from build123d import *

# Parameters (mm, degrees)
SKETCH1_W           = 65
SKETCH1_H           = 159.8
BOSS_EXTRUDE1_DEPTH = 2.5
SKETCH2_W           = 15
SKETCH2_H           = 30
BOSS_EXTRUDE2_DEPTH = 25
SKETCH3_R           = 5.1
CUT_EXTRUDE1_DEPTH  = 107.607973435
SKETCH6_W           = 5
SKETCH6_H           = 5
BOSS_EXTRUDE4_DEPTH = 5
SKETCH7_R           = 5
BOSS_EXTRUDE5_DEPTH = 21
SKETCH8_R           = 15
BOSS_EXTRUDE6_DEPTH = 3
FILLET1_R           = 1.5
CHAMFER1_SIZE       = 1.5
FILLET2_R           = 1.5


with BuildPart() as part:
    # Sketch1 → Boss-Extrude1 (new, symmetric)
    with BuildSketch(Plane(origin=(0, 0, 0), x_dir=(1, 0, 0), z_dir=(0, 1, 0))):
        Rectangle(SKETCH1_W, SKETCH1_H)
    extrude(amount=BOSS_EXTRUDE1_DEPTH, both=True)

    # Sketch2 → Boss-Extrude2 (add)
    with BuildSketch(Plane(origin=(0, 2.5, 0), x_dir=(1, 0, 0), z_dir=(0, 1, 0))):
        with Locations((-25, 0)):
            Rectangle(SKETCH2_W, SKETCH2_H)
    extrude(amount=BOSS_EXTRUDE2_DEPTH)

    # Sketch3 → Cut-Extrude1 (cut, through all)
    with BuildSketch(Plane.ZY.offset(32.5)):
        with Locations((0, 15)):
            Circle(SKETCH3_R)
    extrude(amount=-CUT_EXTRUDE1_DEPTH, mode=Mode.SUBTRACT)

    # Sketch6 → Boss-Extrude4 (add)
    with BuildSketch(Plane.XZ.offset(2.5)):
        with Locations((30, 77.4)):
            Rectangle(SKETCH6_W, SKETCH6_H)
        with Locations((30, -77.4)):
            Rectangle(SKETCH6_W, SKETCH6_H)
    extrude(amount=BOSS_EXTRUDE4_DEPTH)

    # Sketch7 → Boss-Extrude5 (add)
    with BuildSketch(Plane(origin=(0, 2.5, 0), x_dir=(1, 0, 0), z_dir=(0, 1, 0))):
        with Locations(Location((-11.5, 40, 0), (0, 0, 90))):
            Circle(SKETCH7_R)
        with Locations(Location((-11.5, -40, 0), (0, 0, 90))):
            Circle(SKETCH7_R)
    extrude(amount=BOSS_EXTRUDE5_DEPTH)

    # Sketch8 → Boss-Extrude6 (add)
    with BuildSketch(Plane(origin=(0, 23.5, 0), x_dir=(1, 0, 0), z_dir=(0, 1, 0))):
        with Locations(Location((-11.5, 40, 0), (0, 0, 270))):
            Circle(SKETCH8_R)
        with Locations(Location((-11.5, -40, 0), (0, 0, 90))):
            Circle(SKETCH8_R)
    extrude(amount=BOSS_EXTRUDE6_DEPTH)

    # Fillet1
    fillet1_edges = [part.edges().sort_by_distance(p)[0] for p in [
        (-11.5, 23.5, -55),
        (-11.5, 26.5, -55),
        (-11.5, 23.5, 55),
        (-11.5, 26.5, 55),
    ]]
    fillet(fillet1_edges, radius=FILLET1_R - 0.0001)  # a hair under: the kernel refuses the full size

    # Chamfer1
    chamfer1_edges = [part.edges().sort_by_distance(p)[0] for p in [
        (-32.5, 15, -5.1),
    ]]
    chamfer(chamfer1_edges, length=CHAMFER1_SIZE)

    # Fillet2
    fillet2_edges = [part.edges().sort_by_distance(p)[0] for p in [
        (-32.5, 15, -15),
        (-32.5, 15, 15),
        (-17.5, 15, 15),
        (-17.5, 15, -15),
        (-32.5, 27.5, 0),
        (-25, 27.5, 15),
        (-17.5, 27.5, 0),
        (-25, 27.5, -15),
    ]]
    fillet(fillet2_edges, radius=FILLET2_R)


solid = part.part
Can you work these out from the model? Positions are in its coordinate system, mm. A direction names the side the tool comes from. Coordinates: 2 decimals unless noted, no trailing zeros. Loops run counter-clockwise (first coordinate to the right, second up) from the corner with the lowest first, then second, coordinate; pieces in that order, holes last. Notation, with made-up numbers: (4, 63) - (41, 63) arc R25 ccw to (41, 84) - close; hole circle Ø10 at (66.5, 0). An arc over 180 degrees is marked (long way). Put each result on its own line as item: value. Start each with the question number.
Item 1: Which directions (+Z, -Z, +X, -X, +Y, -Y) give clear straight access to the entire face, cutting with the end or side of a thin tool? Please do faces 5 (the face through (30, -5, 74.9)), 6 (the face through (-11, 26.5, -40)), 7 (the face through (32.5, 0, -1)), 8 (the face through (27.5, -5, 77)), 9 (the face through (-6, 23.5, 40)).
Item 2: If we mould it in two halves opening along Y, with no side actions, what happens to faces 1 (the face through (-24, 10, -1)), 2 (the face through (-25, 27.5, 0)), 3 (the face through (0, 0, 79.9)), 4 (the face through (30, -7.5, -77))? For each: +Y half, -Y half, draft (parallel to the pull), parting line (faces both ways), or undercut.
Item 3: If I drill on line 1 along Y through (x, z) = (-20, 0); line 2 along Y through (x, z) = (25, -66.5); line 3 along Z through (x, y) = (-21.5, 24), over which ranges is the centre line in solid material (lowest first)?
Item 4: Suppose I cut it at A-A (y = 15). Please give me the cut outline in (x, z), and give its area (3 significant figures).
Item 5: For pin 1 (13.5 mm diameter, centred on x = -9.5, z = -40, fed in from -Y); pin 2 (8 mm diameter, centred on x = -15.5, z = -39, fed in from +Y); pin 3 (2 mm diameter, centred on x = -19.5, y = 7, fed in from +Z), each with a flat end and sliding along its axis, tell me the tip position at first contact or that it passes through.
Item 6: Suppose I cut it at C-C (y = 5.5). Please give me the cut outline in (x, z).
Here are the results:
1. face 5: +X, -X, -Y
1. face 6: -Z, +X, -X, +Y
1. face 7: +Z, -Z, +X, +Y, -Y
1. face 8: +Z, -Z, -X, -Y
1. face 9: none
2. face 1: undercut
2. face 2: +Y half
2. face 3: draft
2. face 4: -Y half
3. line 1: -2.5 to 9.9, 20.1 to 27.5
3. line 2: -2.5 to 2.5
3. line 3: -50.66 to -29.34, -15 to 15, 29.34 to 50.66
4. outline: (-32.5, -13.5) arc R1.5 ccw to (-31, -15) - (-19, -15) arc R1.5 ccw to (-17.5, -13.5) - (-17.5, -5.1) - (-31, -5.1) - (-32.5, -6.6) - close; (-32.5, 6.6) - (-31, 5.1) - (-17.5, 5.1) - (-17.5, 13.5) arc R1.5 ccw to (-19, 15) - (-31, 15) arc R1.5 ccw to (-32.5, 13.5) - close; circle Ø10 at (-11.5, -40); circle Ø10 at (-11.5, 40)
4. area: 450 mm²
5. pin 1: y = -2.5
5. pin 2: y = 26.5
5. pin 3: z = 15
6. outline: (-32.5, -13.5) arc R1.5 ccw to (-31, -15) - (-19, -15) arc R1.5 ccw to (-17.5, -13.5) - (-17.5, 13.5) arc R1.5 ccw to (-19, 15) - (-31, 15) arc R1.5 ccw to (-32.5, 13.5) - close; circle Ø10 at (-11.5, -40); circle Ø10 at (-11.5, 40)
